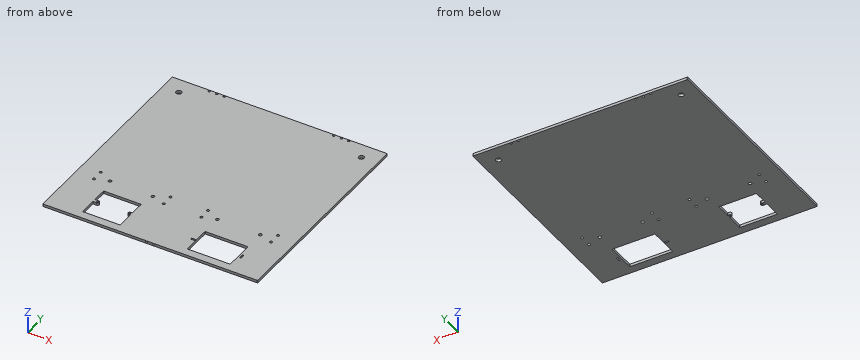
from build123d import *

# Parameters (mm, degrees)
SKETCH1_R           = 2.5
SKETCH1_R_2         = 3
SKETCH1_R_3         = 2
SKETCH1_R_4         = 5.1
BOSS_EXTRUDE1_DEPTH = 5
SKETCH2_R           = 2
CUT_EXTRUDE1_DEPTH  = 8
SKETCH3_R           = 1.5
BOSS_EXTRUDE2_DEPTH = 5


with BuildPart() as part:
    # Sketch1 → Boss-Extrude1 (new body)
    with BuildSketch(Plane.XY):
        with BuildLine():
            Line((1, 0), (399, 0))
            ThreePointArc((399, 0), (399.707106781, 0.292893219), (400, 1))
            Line((400, 1), (400, 399))
            ThreePointArc((400, 399), (399.707106781, 399.707106781), (399, 400))
            Line((399, 400), (1, 400))
            ThreePointArc((1, 400), (0.292893219, 399.707106781), (0, 399))
            Line((0, 399), (0, 1))
            ThreePointArc((0, 1), (0.292893219, 0.292893219), (1, 0))
        make_face()
        with Locations((35, 121)):
            Circle(SKETCH1_R, mode=Mode.SUBTRACT)
        with Locations((35, 100)):
            Circle(SKETCH1_R, mode=Mode.SUBTRACT)
        with Locations((60, 108)):
            Circle(SKETCH1_R_2, mode=Mode.SUBTRACT)
        with Locations((140, 108)):
            Circle(SKETCH1_R_2, mode=Mode.SUBTRACT)
        with Locations((165, 121)):
            Circle(SKETCH1_R, mode=Mode.SUBTRACT)
        with Locations((165, 100)):
            Circle(SKETCH1_R, mode=Mode.SUBTRACT)
        with Locations((235, 121)):
            Circle(SKETCH1_R, mode=Mode.SUBTRACT)
        with Locations((235, 100)):
            Circle(SKETCH1_R, mode=Mode.SUBTRACT)
        with Locations((260, 108)):
            Circle(SKETCH1_R_2, mode=Mode.SUBTRACT)
        with Locations((340, 108)):
            Circle(SKETCH1_R_2, mode=Mode.SUBTRACT)
        with Locations((365, 121)):
            Circle(SKETCH1_R, mode=Mode.SUBTRACT)
        with Locations((365, 100)):
            Circle(SKETCH1_R, mode=Mode.SUBTRACT)
        with Locations((70, 397.5)):
            Circle(SKETCH1_R_3, mode=Mode.SUBTRACT)
        with Locations((84, 397.5)):
            Circle(SKETCH1_R_3, mode=Mode.SUBTRACT)
        with Locations((98, 397.5)):
            Circle(SKETCH1_R_3, mode=Mode.SUBTRACT)
        with Locations((302, 397.5)):
            Circle(SKETCH1_R_3, mode=Mode.SUBTRACT)
        with Locations((316, 397.5)):
            Circle(SKETCH1_R_3, mode=Mode.SUBTRACT)
        with Locations((330, 397.5)):
            Circle(SKETCH1_R_3, mode=Mode.SUBTRACT)
        with Locations((30, 370)):
            Circle(SKETCH1_R_4, mode=Mode.SUBTRACT)
        with Locations((370, 370)):
            Circle(SKETCH1_R_4, mode=Mode.SUBTRACT)
        with BuildLine():
            Line((261, 70), (339, 70))
            ThreePointArc((339, 70), (339.707106781, 69.707106781), (340, 69))
            Line((340, 69), (340, 16))
            ThreePointArc((340, 16), (339.707106781, 15.292893219), (339, 15))
            Line((339, 15), (261, 15))
            ThreePointArc((261, 15), (260.292893219, 15.292893219), (260, 16))
            Line((260, 16), (260, 69))
            ThreePointArc((260, 69), (260.292893219, 69.707106781), (261, 70))
        make_face(mode=Mode.SUBTRACT)
        with BuildLine():
            Line((66, 80), (134, 80))
            ThreePointArc((134, 80), (134.707106781, 79.707106781), (135, 79))
            Line((135, 79), (135, 16))
            ThreePointArc((135, 16), (134.707106781, 15.292893219), (134, 15))
            Line((134, 15), (66, 15))
            ThreePointArc((66, 15), (65.292893219, 15.292893219), (65, 16))
            Line((65, 16), (65, 79))
            ThreePointArc((65, 79), (65.292893219, 79.707106781), (66, 80))
        make_face(mode=Mode.SUBTRACT)
        with BuildLine():
            Line((346.5, 45), (346.5, 39))
            ThreePointArc((346.5, 39), (345, 37.5), (343.5, 39))
            Line((343.5, 39), (343.5, 45))
            ThreePointArc((343.5, 45), (345, 46.5), (346.5, 45))
        make_face(mode=Mode.SUBTRACT)
        with BuildLine():
            Line((252, 43.5), (258, 43.5))
            ThreePointArc((258, 43.5), (259.5, 42), (258, 40.5))
            Line((258, 40.5), (252, 40.5))
            ThreePointArc((252, 40.5), (250.5, 42), (252, 43.5))
        make_face(mode=Mode.SUBTRACT)
    extrude(amount=BOSS_EXTRUDE1_DEPTH)

    # Sketch2 → Cut-Extrude1 (cut)
    with BuildSketch(Plane.XZ):
        with Locations(Location((193, 2.5, 0), (0, 0, 270))):
            Circle(SKETCH2_R)
        with Locations(Location((207, 2.5, 0), (0, 0, 270))):
            Circle(SKETCH2_R)
    extrude(amount=-CUT_EXTRUDE1_DEPTH, mode=Mode.SUBTRACT)

    # Sketch3 → Boss-Extrude2 (add)
    # profile 1 of 2: a face of its own
    with BuildSketch(Plane.XY):
        with BuildLine():
            Line((132, 53), (135, 53))
            Line((135, 53), (135, 47))
            Line((135, 47), (132, 47))
            ThreePointArc((132, 47), (129, 50), (132, 53))
        make_face()
        with Locations((132, 50)):
            Circle(SKETCH3_R, mode=Mode.SUBTRACT)
    # profile 2 of 2: a face of its own
    with BuildSketch(Plane.XY):
        with BuildLine():
            Line((72, 47), (65, 47))
            Line((65, 47), (65, 53))
            Line((65, 53), (72, 53))
            ThreePointArc((72, 53), (75, 50), (72, 47))
        make_face()
        with Locations((72, 50)):
            Circle(SKETCH3_R, mode=Mode.SUBTRACT)
    extrude(amount=BOSS_EXTRUDE2_DEPTH)


solid = part.part
For this review, take the finished solid that the model builds, in its own axes (mm). Give positions to 0.01 mm unless a question says otherwise; leave off trailing zeros. Order: outer loops, then holes, each group sorted by start corner. A loop starts at its lowest first (then second) coordinate and runs counter-clockwise, first axis right, second up. Notation, with made-up numbers: (50.25, 24) - (98.25, 24) arc R9 ccw to (98.25, 32) - close; hole circle Ø9 at (54.5, -8). An arc over 180 degrees is marked (long way). Answer as a JSON object with one key per item and string values. Group by question number.
Item 1: Take a section at A-A on x = 118.5. Give the boundary of the cut face in (y, z).
Item 2: Wall thickness on line 1 along Y through (x, z) = (132, 2.15); line 2 along Y through (x, z) = (235, 3); line 3 along Y through (x, z) = (140, 1.9): over which ranges is each line inside the solid? List them lowest first.
Item 3: Take a section at B-B on z = 2.9. Give the number of separate pieces and of enclosed holes in the cut face, and give its area (3 significant figures).
Item 4: Clearance check with flat-ended pins moving along their axes: pin 1 Ø4 at (x, y) = (35, 121) entering from -Z; pin 2 Ø1.2 at (x, z) = (193, 2) entering from -Y. State where each tip first meets the part, or that it passes through.
Reported:
{
 "1": {"outline": "(0, 0) - (15, 0) - (15, 5) - (0, 5) - close; (80, 0) - (400, 0) - (400, 5) - (80, 5) - close"},
 "2": {"line 1": "0 to 15, 47 to 48.5, 51.5 to 53, 80 to 400", "line 2": "0 to 97.5, 102.5 to 118.5, 123.5 to 400", "line 3": "0 to 105, 111 to 400"},
 "3": {"separate pieces": "1", "enclosed holes": "26", "area": "151,000 mm^2"},
 "4": {"pin 1": "through", "pin 2": "y = 8"}
}
